Autodesk Inventor part; units mm, degrees
ref_plane "YZ Plane" through (0, 0, 0) normal (1, 0, 0) x (0, 1, 0)
ref_plane "XZ Plane" through (0, 0, 0) normal (0, 1, 0) x (-1, 0, 0)
ref_plane "XY Plane" through (0, 0, 0) normal (0, 0, 1) x (1, 0, 0)
sketch "Sketch3" plane through (0, 0, 0) normal (1, 0, 0) x (0, 1, 0)
  circle A0 centre (0, 0) radius 1.5
  arc A1 (1.725, -2.4545) -> (-1.6531, -2.5034) centre (0, 0) ccw
  line L0 (-0.7552, -4.1724) -> (-0.7552, -10)
  line L1 (-0.7552, -10) -> (0.875, -10)
  line L2 (0.875, -10) -> (0.875, -4.0908)
  arc A2 (1.725, -2.4545) -> (0.875, -4.0908) centre (2.875, -4.0908) ccw
  arc A3 (-0.7552, -4.1724) -> (-1.6531, -2.5034) centre (-2.7552, -4.1724) ccw
  dimension "d4" = 3
  dimension "d5" = 6
  dimension "d7" = 2
extrude "Extrusion2" add sketch "Sketch3" along normal blind 30
sketch "Sketch5" plane through (0, 0.875, -4.0908) normal (0, 1, 0) x (1, 0, 0)
  line L0 (0, 5.9092) -> (30, 5.9092)
  line L1 (6, 5.9092) -> (24, 5.9092)
  line L2 (24, 5.9092) -> (24, -0.0908)
  line L3 (24, -0.0908) -> (6, -0.0908)
  line L4 (6, -0.0908) -> (6, 5.9092)
  line L5 (0, 5.9092) -> (0, 0)
  point P0 (0, -4.0908)
  dimension "d18" = 6
  dimension "d19" = 30
  dimension "d20" = 6
  dimension "d21" = 18
extrude "Extrusion3" cut sketch "Sketch5" along normal blind 0.5 and the other way blind 2
fillet "Fillet1" radius 2 6 edges at (6, 0.0599, -10) (24, 0.0599, -10) (30, 0.0599, -10) (0, 0.0599, -10) (24, 0.0572, -4) (6, 0.0572, -4)
chamfer "Chamfer2" distance 0.25 angle 45 38 edges at (5.4142, 0.875, -9.4142) (6, 0.875, -7) (6.3889, 0.875, -4.815) (7.6998, 0.8762, -4.0227) (15, 0.8771, -4) (22.3002, 0.8762, -4.0227) (23.6111, 0.875, -4.815) (24, 0.875, -7) (24.5858, 0.875, -9.4142) (27, 0.875, -10) (29.4142, 0.875, -9.4142) (30, 0.875, -6.0454) (30, 1.1002, -3.1688) (30, -0.0435, 2.9997) (30, -0.9939, -3.2248) (30, -0.7552, -6.0862) (29.4142, -0.7552, -9.4142) (27, -0.7552, -10) (24.5858, -0.7552, -9.4142) (24, -0.7552, -7) (23.677, -0.7552, -4.9102) (22.4123, -0.7594, -4.043) (15, -0.7626, -4) (7.5877, -0.7594, -4.043) (6.323, -0.7552, -4.9102) (6, -0.7552, -7) (5.4142, -0.7552, -9.4142) (3, -0.7552, -10) (0.5858, -0.7552, -9.4142) (0, -0.7552, -6.0862) (0, -0.9939, -3.2248) (0, -0.0435, 2.9997) (0, 1.1002, -3.1688) (0, 0.875, -6.0454) (0.5858, 0.875, -9.4142) (3, 0.875, -10) (30, -1.5, 0) (0, -1.5, 0)
equation "\"d20\" = -0.5 * d21 + 0.5 * d19"
properties part number "CoinLockUpperRow"
Could you check a few things on this model? Use its own coordinates, in mm. A direction names the side the tool comes from. Give positions to 0.01 mm unless a question says otherwise; leave off trailing zeros. Use one line per item in the form item = value.
1. I need wall thicknesses on probe 1 along Y at (x, z) = (27.5, -5) (3 decimals); probe 2 along Y at (x, z) = (2, -0.5); probe 3 along Z at (x, y) = (14.5, 0). Which ranges of each line are inside material? Lowest first, please.
Response values:
probe_1 = -0.755 to 0.875
probe_2 = -2.96 to -1.41, 1.41 to 2.96
probe_3 = -4 to -1.5, 1.5 to 3
2. Thinking about a two-plate mould opening in Y: for faces 1 (the face through (14.79, -1.5, -0.07)), 2 (the face through (29.43, 0.07, -9.4)), 3 (the face through (5.34, -0.63, -9.31)), which applies, released by +Y, released by -Y, zero draft, split by the parting line, or undercut?
Response values:
face_1 = undercut
face_2 = zero draft
face_3 = released by -Y
3. On a 3-axis mill with a long thin cutter (end or side, diameter ignored), from which of +Z, -Z, +X, -X, +Y, -Y can I reach the whole of each face in a straight line? I mean faces 4 (the face through (3, -0.755, -7)), 5 (the face through (24.66, 0.75, -9.31)), 6 (the face through (24, 0, -7)). Say none if no direction works.
Response values:
face_4 = -Z, +X, -X, -Y
face_5 = -Z, +Y
face_6 = -Z, +Y, -Y
4. I'm going to push flat-ended pins straight in: pin 1 Ø1 at (x, y) = (4.5, 0.5) entering from -Z; pin 2 Ø1.3 at (x, y) = (14.5, 0.5) entering from -Z; pin 3 Ø1.8 at (y, z) = (0, 0) entering from -X; pin 4 Ø1 at (x, y) = (11, -2) entering from -Z. Where does each tip first touch, or does it pass through?
Response values:
pin_1 = -10
pin_2 = -4
pin_3 = through
pin_4 = -2.62
